Build history of the part. All positions in model axes, mm. Round coordinates to 2 decimals unless told otherwise and drop trailing zeros. Write each loop counter-clockwise with the first axis right and the second up, starting at its lowest first coordinate (ties: lowest second). Pieces come first, ordered by that corner, then holes. Notation, with made-up numbers: (18, 77) - (39, 77) arc R37 ccw to (39, 114) - close; hole circle Ø6 at (44.5, -13.75). An arc over 180 degrees is marked (long way). Answer as a JSON object with one key per item and string values. Group by question number.
Item 1: Slice it at D-D, the plane x = -1.25. List the corners of the cut face in (y, z), then the cut area to 3 significant figures.
Item 2: Slice it at B-B, the plane z = 15.75. List the corners of the cut face in (x, y), then the cut area to 3 significant figures.
Item 3: Probe line 1 (Y direction, x = -7.75, z = 9); line 2 (X direction, y = -2.25, z = 10.75); line 3 (Y direction, x = 8.25, z = 12). List the from-to ranges inside material, lowest first. Write a range as from..to.
Item 4: Flat gauge pins, fed straight in: pin 1 (0.8 mm diameter, centred on y = -1.5, z = 16.5, fed in from -X); pin 2 (1 mm diameter, centred on y = -2.5, z = 14, fed in from +X). Where does each tip first touch, or does it go through?
Item 5: Slice it at A-A, the plane y = -2.05. List the corners of the cut face in (x, z).
Item 6: Slice it at C-C, the plane x = -4.5. List the corners of the cut face in (y, z), then the cut area to 3 significant figures.
from build123d import *

# Parameters (mm, degrees)
BOSS_EXTRUDE1_DEPTH = 25
BOSS_EXTRUDE2_DEPTH = 1
FILLET1_R           = 0.3
FILLET2_R           = 0.3


with BuildPart() as part:
    # Sketch1 → Boss-Extrude1 (new body)
    with BuildSketch(Plane.XY):
        Polygon((8, -1), (8, -2.5), (9, -3.5), (9, -4.5), (-9, -4.5), (-9, -3.5), (-8, -2.5), (-8, -1), (-9, -1), (-9, 0), (9, 0), (9, -1), align=None)
    extrude(amount=BOSS_EXTRUDE1_DEPTH)

    # Sketch2 → Boss-Extrude2 (add)
    with BuildSketch(Plane(origin=(0, 0, 0), x_dir=(1, 0, 0), z_dir=(0, 1, 0))):
        with BuildLine():
            Line((6, -3.5), (6, -21.5))
            ThreePointArc((6, -21.5), (4.5, -23), (3, -21.5))
            Line((3, -21.5), (3, -3.5))
            ThreePointArc((3, -3.5), (4.5, -2), (6, -3.5))
        make_face()
        with BuildLine():
            Line((-6, -3.5), (-6, -21.5))
            ThreePointArc((-6, -21.5), (-4.5, -23), (-3, -21.5))
            Line((-3, -21.5), (-3, -3.5))
            ThreePointArc((-3, -3.5), (-4.5, -2), (-6, -3.5))
        make_face()
    extrude(amount=BOSS_EXTRUDE2_DEPTH)

    # Fillet1
    fillet1_edges = [part.edges().sort_by_distance(p)[0] for p in [
        (4.5, 0, 2),
        (3, 0, 12.5),
        (4.5, 0, 23),
        (6, 0, 12.5),
        (4.5, 1, 2),
        (3, 1, 12.5),
        (4.5, 1, 23),
        (6, 1, 12.5),
        (-4.5, 0, 2),
        (-6, 0, 12.5),
        (-4.5, 0, 23),
        (-3, 0, 12.5),
        (-4.5, 1, 2),
        (-6, 1, 12.5),
        (-4.5, 1, 23),
        (-3, 1, 12.5),
    ]]
    fillet(fillet1_edges, radius=FILLET1_R)

    # Fillet2
    fillet2_edges = [part.edges().sort_by_distance(p)[0] for p in [
        (8, -1.75, 0),
        (8.5, -3, 0),
        (0, 0, 25),
        (9, -4, 0),
        (0, -4.5, 0),
        (-9, -4, 0),
        (-8.5, -3, 0),
        (-8, -1.75, 0),
        (-8.5, -1, 0),
        (-9, -0.5, 0),
        (0, 0, 0),
        (9, -0.5, 0),
        (8.5, -1, 0),
        (-9, -0.5, 25),
        (-8.5, -1, 25),
        (-8, -1.75, 25),
        (-8.5, -3, 25),
        (-9, -4, 25),
        (0, -4.5, 25),
        (9, -4, 25),
        (8.5, -3, 25),
        (8, -1.75, 25),
        (8.5, -1, 25),
        (9, -0.5, 25),
    ]]
    fillet(fillet2_edges, radius=FILLET2_R)


solid = part.part
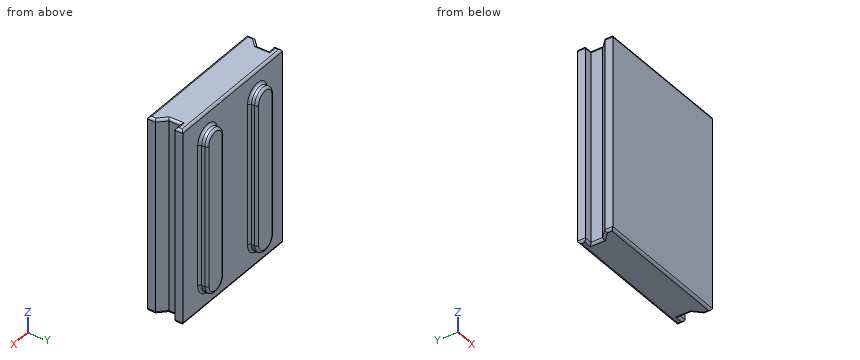
Geometry says:
{
 "1": {"outline": "(-4.5, 0.3) arc R0.3 ccw to (-4.2, 0) - (-0.3, 0) arc R0.3 ccw to (0, 0.3) - (0, 24.7) arc R0.3 ccw to (-0.3, 25) - (-4.2, 25) arc R0.3 ccw to (-4.5, 24.7) - close", "area": "112 mm^2"},
 "2": {"outline": "(-9, -4.5) - (9, -4.5) - (9, -3.5) - (8, -2.5) - (8, -1) - (9, -1) - (9, 0) - (6.3, 0) arc R0.3 cw to (6, 0.3) - (6, 0.7) arc R0.3 ccw to (5.7, 1) - (3.3, 1) arc R0.3 ccw to (3, 0.7) - (3, 0.3) arc R0.3 cw to (2.7, 0) - (-2.7, 0) arc R0.3 cw to (-3, 0.3) - (-3, 0.7) arc R0.3 ccw to (-3.3, 1) - (-5.7, 1) arc R0.3 ccw to (-6, 0.7) - (-6, 0.3) arc R0.3 cw to (-6.3, 0) - (-9, 0) - (-9, -1) - (-8, -1) - (-8, -2.5) - (-9, -3.5) - close", "area": "83.0 mm^2"},
 "3": {"line 1": "y = -4.5..0", "line 2": "x = -8..8", "line 3": "y = -4.5..-2.75, -1..0"},
 "4": {"pin 1": "stops at x = -8", "pin 2": "stops at x = 8.5"},
 "5": {"outline": "(-8, 0.3) arc R0.3 ccw to (-7.7, 0) - (7.7, 0) arc R0.3 ccw to (8, 0.3) - (8, 24.7) arc R0.3 ccw to (7.7, 25) - (-7.7, 25) arc R0.3 ccw to (-8, 24.7) - close"},
 "6": {"outline": "(-4.5, 0.3) arc R0.3 ccw to (-4.2, 0) - (-0.3, 0) arc R0.3 ccw to (0, 0.3) - (0, 1.7) arc R0.3 cw to (0.3, 2) - (0.7, 2) arc R0.3 ccw to (1, 2.3) - (1, 22.7) arc R0.3 ccw to (0.7, 23) - (0.3, 23) arc R0.3 cw to (0, 23.3) - (0, 24.7) arc R0.3 ccw to (-0.3, 25) - (-4.2, 25) arc R0.3 ccw to (-4.5, 24.7) - close", "area": "133 mm^2"}
}
